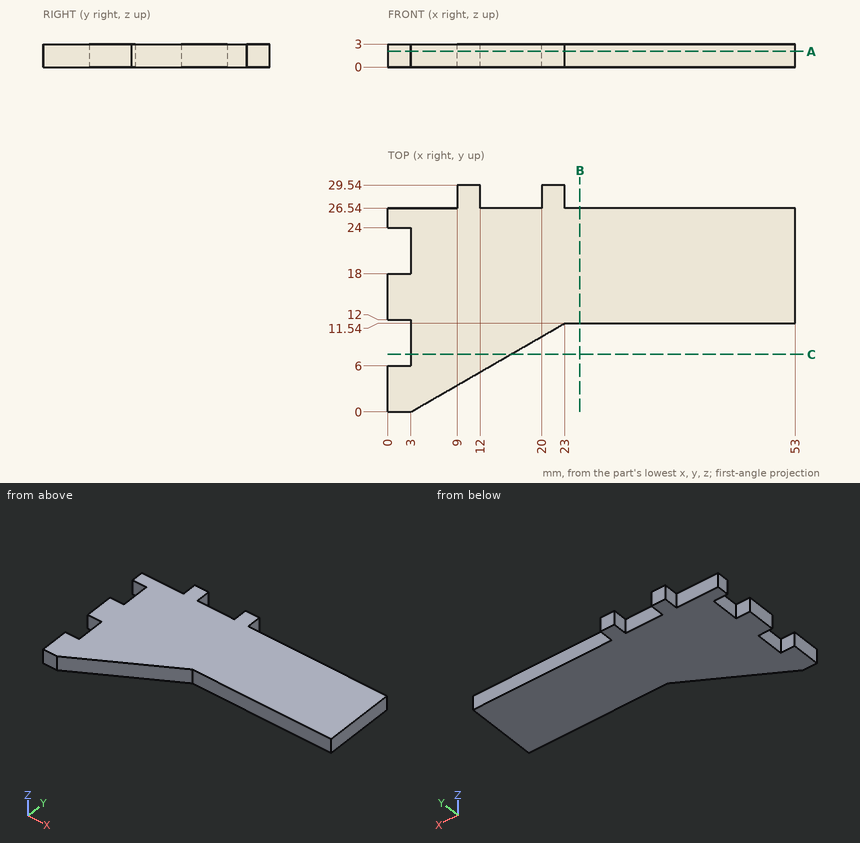
Input: dimensioned drawing with shaded views. Units: mm. Origin: part minimum x, y, z. Coordinates: 2 decimals unless noted, no trailing zeros. Loops run counter-clockwise (first coordinate to the right, second up) from the corner with the lowest first, then second, coordinate; pieces in that order, holes last. Notation, with made-up numbers: (57.5, 14) -> (76.5, 14) arc R23 cw to (76.5, 26) -> close; hole circle Ø11 at (0.5, 76.25). An arc over 180 degrees is marked (long way). Use a Markdown table: item, result. Add a question column.
(1) Section query B-B, the plane x = 25. Return loops of the section in (y, z), plus the area to 3 significant figures.
(2) Line query: line 1 along Y through (x, z) = (2, 1.4); line 2 along X through (y, z) = (27.25, 1.4); line 3 along Y through (x, z) = (24.5, 0.7). Output: solid intervals per line, ascending.
(3) Section query C-C, the plane y = 7.5. Return loops of the section in (x, z), plus the area to 3 significant figures.
(4) Section query A-A, the plane z = 2.05. Return loops of the section in (x, y).
(5) Pin query (flat end, axial travel): pin 1 Ø0.9 at (y, z) = (20.5, 1) entering from -X; pin 2 Ø0.9 at (x, z) = (41, 2) entering from +Y; pin 3 Ø0.9 at (y, z) = (28, 2) entering from -X. Return the tip coordinate at first contact, or that it passes through.
Answer:
| question | item | result |
|---|---|---|
| 1 | outline | (11.54, 0) -> (26.54, 0) -> (26.54, 3) -> (11.54, 3) -> close |
| 1 | area | 45.0 mm^2 |
| 2 | line 1 | y = 0 to 6, 12 to 18, 24 to 26.54 |
| 2 | line 2 | x = 9 to 12, 20 to 23 |
| 2 | line 3 | y = 11.54 to 26.54 |
| 3 | outline | (3, 0) -> (16, 0) -> (16, 3) -> (3, 3) -> close |
| 3 | area | 39.0 mm^2 |
| 4 | outline | (0, 0) -> (3, 0) -> (23, 11.54) -> (53, 11.54) -> (53, 26.54) -> (23, 26.54) -> (23, 29.54) -> (20, 29.54) -> (20, 26.54) -> (12, 26.54) -> (12, 29.54) -> (9, 29.54) -> (9, 26.54) -> (0, 26.54) -> (0, 24) -> (3, 24) -> (3, 18) -> (0, 18) -> (0, 12) -> (3, 12) -> (3, 6) -> (0, 6) -> close |
| 5 | pin 1 | stops at x = 3 |
| 5 | pin 2 | stops at y = 26.54 |
| 5 | pin 3 | stops at x = 9 |
